Design review of the part built by this model. Coordinates are the model's own, in mm. A direction names the side the tool comes from. Coordinates: 2 decimals unless noted, no trailing zeros. Write each loop counter-clockwise with the first axis right and the second up, starting at its lowest first coordinate (ties: lowest second). Pieces come first, ordered by that corner, then holes. Notation, with made-up numbers: M 88.5,84.25 L 101.5,84.25 A8 ccw 101.5,89.25 Z; hole C -30.75,3.25 d4. An arc over 180 degrees is marked long. Return JSON: item names as keys, results as strings. Group by question number.
Autodesk Inventor part; units mm, degrees
ref_plane "YZ Plane" through (0, 0, 0) normal (1, 0, 0) x (0, 1, 0)
ref_plane "XZ Plane" through (0, 0, 0) normal (0, 1, 0) x (-1, 0, 0)
ref_plane "XY Plane" through (0, 0, 0) normal (0, 0, 1) x (1, 0, 0)
sketch "スケッチ1" plane through (0, 0, 0) normal (0, 0, 1) x (1, 0, 0)
  circle A0 centre (0, 0) radius 2.75
  dimension "d0" = 5.5
extrude "押し出し1" add sketch "スケッチ1" along normal blind 3
sketch "スケッチ2" plane through (0, 0, 0) normal (0, 0, -1) x (-1, 0, 0)
  circle A0 centre (0, 0) radius 2.75
  circle A1 centre (0, 0) radius 1.5
  dimension "d3" = 3
extrude "押し出し2" add sketch "スケッチ2" along normal blind 6 contours A1
sketch "スケッチ3" plane through (0, 0, 3) normal (0, 0, 1) x (1, 0, 0)
  circle A0 centre (0, 0) radius 2.75
  line L0 (0, 1.4434) -> (1.25, 0.7217)
  line L1 (1.25, 0.7217) -> (1.25, -0.7217)
  line L2 (1.25, -0.7217) -> (0, -1.4434)
  line L3 (0, -1.4434) -> (-1.25, -0.7217)
  line L4 (-1.25, -0.7217) -> (-1.25, 0.7217)
  line L5 (-1.25, 0.7217) -> (0, 1.4434)
  dimension "d6" = 1.25
extrude "押し出し3" cut sketch "スケッチ3" against normal blind 1.5 contours L0 L1 L2 L3 L4 L5
fillet "フィレット1" radius 0.5 2 edges at (-2.75, 0, 3) (-2.75, 0, 0)
fillet "フィレット2" radius 0.3 19 edges at (-0.625, 1.0825, 3) (-1.25, 0, 3) (-0.625, -1.0825, 3) (0.625, -1.0825, 3) (1.25, 0, 3) (0.625, 1.0825, 3) (-0.625, 1.0825, 1.5) (0.625, 1.0825, 1.5) (0, 1.4434, 2.25) (-1.25, 0.7217, 2.25) (-0.625, -1.0825, 1.5) (-1.25, -0.7217, 2.25) (-1.25, 0, 1.5) (1.25, 0, 1.5) (1.25, 0.7217, 2.25) (1.25, -0.7217, 2.25) (0.625, -1.0825, 1.5) (0, -1.4434, 2.25) (1.5, 0, -6)
thread "ねじ2"
Item 1: Machinability: for faces 1 (the flat face through (0, 0, -6)), 2 (the flat face through (0.618, 1.086, 2.256)), 3 (the flat face through (-2, 0, 0)), which of the approach directions +Z, -Z, +X, -X, +Y, -Y give a long, thin tool a straight path to every point of the face, cutting with its end or side? Answer none if there is none.
Item 2: Add section C-C (z = -2.5). Write out the cut boundary in (x, y), plus the area to 3 significant figures.
Item 3: For pin 1 (2 mm diameter, centred on x = 0, y = -0.5, fed in from +Z); pin 2 (1 mm diameter, centred on x = 2, y = 0.5, fed in from -Z), all flat-tipped, find the tip position at first contact; note any pin that passes through.
Item 4: The part is to be moulded in two halves that separate along X. For faces 4 (the cylindrical face through (-0.677, -1.157, 2.914)), 5 (the cylindrical face through (-0.596, 2.685, 1.486)), 6 (the flat face through (0, 2, 3)), 7 (the flat face through (-0.618, -1.086, 2.256)), say which applies: pulls with the +X half, pulls with the -X half, needs draft (parallel to the pull), parting line crosses it, or undercut.
Item 5: Add section A-A (y = 0). Write out the cut boundary in (x, z), plus the area to 3 significant figures.
Item 6: Add section B-B (z = 2). Write out the cut boundary in (x, y), plus the area to 3 significant figures.
Item 7: For line 1 (Z direction, x = 0.35, y = -0.5); line 2 (Z direction, x = 2, y = -0.3); line 3 (Y direction, x = -0.05, z = -2), list the stretches that pass through material, from the lowest coordinate up.
Geometry check:
{
 "1": {"face 1": "-Z, +X, -X, +Y, -Y", "face 2": "+Z", "face 3": "-Z"},
 "2": {"outline": "C 0,0 d3", "area": "7.07 mm^2"},
 "3": {"pin 1": "z = 2.98", "pin 2": "z = 0"},
 "4": {"face 4": "undercut", "face 5": "parting line crosses it", "face 6": "needs draft", "face 7": "undercut"},
 "5": {"outline": "M -2.75,0.5 A0.5 ccw -2.25,0 L -1.5,0 L -1.5,-5.7 A0.3 ccw -1.2,-6 L 1.2,-6 A0.3 ccw 1.5,-5.7 L 1.5,0 L 2.25,0 A0.5 ccw 2.75,0.5 L 2.75,2.5 A0.5 ccw 2.25,3 L 1.55,3 A0.3 ccw 1.25,2.7 L 1.25,1.8 A0.3 cw 0.95,1.5 L -0.95,1.5 A0.3 cw -1.25,1.8 L -1.25,2.7 A0.3 ccw -1.55,3 L -2.25,3 A0.5 ccw -2.75,2.5 Z", "area": "30.5 mm^2"},
 "6": {"outline": "C 0,0 d5.5; hole M -1.25,-0.55 A0.3 ccw -1.1,-0.81 L -0.15,-1.36 A0.3 ccw 0.15,-1.36 L 1.1,-0.81 A0.3 ccw 1.25,-0.55 L 1.25,0.55 A0.3 ccw 1.1,0.81 L 0.15,1.36 A0.3 ccw -0.15,1.36 L -1.1,0.81 A0.3 ccw -1.25,0.55 Z", "area": "18.4 mm^2"},
 "7": {"line 1": "-6 to 1.5", "line 2": "0 to 3", "line 3": "-1.5 to 1.5"}
}
